Geometry check sheet. Reference: the model listing, model coordinates, mm. A direction names the side the tool comes from. Give positions to 0.01 mm unless a question says otherwise; leave off trailing zeros. Loops run counter-clockwise (first coordinate to the right, second up) from the corner with the lowest first, then second, coordinate; pieces in that order, holes last. Notation, with made-up numbers: (79, 20.25) -> (113, 20.25) arc R15 cw to (113, 35.25) -> close; hole circle Ø5 at (75, -18). An arc over 180 degrees is marked (long way). Write item = value, one per line.
```python
from build123d import *

# Parameters (mm, degrees)
F0_R     = 1.75
F1_DEPTH = 3
F2_R     = 12.25
F3_DEPTH = 2


with BuildPart() as f1:
    # F0 (on Top) → F1 (new body)
    with BuildSketch(Plane.XY):
        with BuildLine():
            Line((24.927017, -9.39162), (4.330127, 26.283241))
            ThreePointArc((4.330127, 26.283241), (0, 28.783241), (-4.330127, 26.283241))
            Line((-4.330127, 26.283241), (-24.927017, -9.39162))
            ThreePointArc((-24.927017, -9.39162), (-24.927017, -14.39162), (-20.59689, -16.89162))
            Line((-20.59689, -16.89162), (20.59689, -16.89162))
            ThreePointArc((20.59689, -16.89162), (24.927017, -14.39162), (24.927017, -9.39162))
        make_face()
        with Locations((-20.75, -11.980018)):
            Circle(F0_R, mode=Mode.SUBTRACT)
        with Locations((20.75, -11.980018)):
            Circle(F0_R, mode=Mode.SUBTRACT)
        with Locations((0, 23.960036)):
            Circle(F0_R, mode=Mode.SUBTRACT)
    extrude(amount=F1_DEPTH)

    # F2 (on face) → F3 (join)
    with BuildSketch(Plane.XY.offset(3)):
        Circle(F2_R)
    extrude(amount=F3_DEPTH)


solid = f1.part
```
Item 1: Thickness scan on L1, parallel to X at y = -12, z = 1; L2, parallel to X at y = -11, z = 2.35; L3, parallel to Z at x = 10, y = 13.5. Record the ranges inside material, lowest first. Write a range as [from, to].
Answer:
L1 = [-25.6, -22.5], [-19, 19], [22.5, 25.6]
L2 = [-25.52, -22.2], [-19.3, 19.3], [22.2, 25.52]
L3 = [0, 3]
Item 2: Section check D-D, the plane x = 7. Record the cut outline in (y, z).
Answer:
outline = (-16.89, 0) -> (21.66, 0) -> (21.66, 3) -> (10.05, 3) -> (10.05, 5) -> (-10.05, 5) -> (-10.05, 3) -> (-16.89, 3) -> close
Item 3: Section check C-C, the plane z = 1.9. Record the cut outline in (x, y).
Answer:
outline = (-24.93, -9.39) arc R5 ccw to (-20.6, -16.89) -> (20.6, -16.89) arc R5 ccw to (24.93, -9.39) -> (4.33, 26.28) arc R5 ccw to (-4.33, 26.28) -> close; hole circle Ø3.5 at (-20.75, -11.98); hole circle Ø3.5 at (0, 23.96); hole circle Ø3.5 at (20.75, -11.98)
Item 4: Draft check along X on faces 3 (the cylindrical face through (0.073, 28.783, 1.479)), 4 (the flat face through (14.77, 8.2, 1.48)), 5 (the cylindrical face through (-22.14, -13.04, 1.48)), 6 (the cylindrical face through (19.36, -13.04, 1.48)). Enter one of: +X half, -X half, draft (parallel to the pull), parting line (faces both ways), or undercut.
Answer:
face_3 = parting line
face_4 = +X half
face_5 = undercut
face_6 = undercut
Item 5: Section check A-A, the plane x = 0. Record the cut outline in (y, z).
Answer:
outline = (-16.89, 0) -> (22.21, 0) -> (22.21, 3) -> (12.25, 3) -> (12.25, 5) -> (-12.25, 5) -> (-12.25, 3) -> (-16.89, 3) -> close; (25.71, 0) -> (28.78, 0) -> (28.78, 3) -> (25.71, 3) -> close
Item 6: Section check B-B, the plane y = 0. Record the cut outline in (x, z), plus the area to 3 significant figures.
Answer:
outline = (-19.5, 0) -> (19.5, 0) -> (19.5, 3) -> (12.25, 3) -> (12.25, 5) -> (-12.25, 5) -> (-12.25, 3) -> (-19.5, 3) -> close
area = 166 mm^2
Item 7: Tool access check on faces 1 (the cylindrical face through (-0.2, 25.7, 1.5)), 2 (the flat face through (-12, -4, 3)). Record the directions out of +Z, -Z, +X, -X, +Y, -Y that give a thin tool (end or side, any length) a straight path to the whole face; none if there is none.
Answer:
face_1 = +Z, -Z
face_2 = +Z
Item 8: Gauge pin test, flat ends, axial feed: pin 1 (2 mm diameter, centred on x = -13.5, z = 1, fed in from +Y); pin 2 (12 mm diameter, centred on x = 19.5, y = -11.5, fed in from +Z); pin 3 (1.5 mm diameter, centred on x = -9.5, z = 1.5, fed in from +Y). Record the tip position at first contact, or that the pin passes through.
Answer:
pin_1 = 12.13
pin_2 = 3
pin_3 = 18.63
